Verification items for the finished model (mm, model axes). A direction names the side the tool comes from. Round coordinates to 2 decimals unless told otherwise and drop trailing zeros. Order: outer loops, then holes, each group sorted by start corner. A loop starts at its lowest first (then second) coordinate and runs counter-clockwise, first axis right, second up. Notation, with made-up numbers: M 46,6.5 L 66,6.5 A25 cw 66,22.5 Z; hole C 57,36 d8. An arc over 180 degrees is marked long. Use CSV: the item, a comma, the result in double quotes. Start each with the question number.
Q1. Sectioned sample at B-B (z = -4.25). Enter the section's corners in (x, y) (3 decimals), and give its area (3 significant figures).
Q2. Gauge pin test, flat ends, axial feed: pin 1 Ø2 at (y, z) = (231.5, -5.5) entering from -X; pin 2 Ø3 at (x, z) = (-5.5, -6.5) entering from +Y; pin 3 Ø3 at (x, z) = (-3, -4.5) entering from +Y. Record the tip position at first contact, or that the pin passes through.
Q3. Sectioned sample at C-C (y = 349.5). Enter the section's corners in (x, z).
Q4. Scan lines: line 1 (Y direction, x = 0, z = -1); line 2 (Y direction, x = -0.75, z = -4.25); line 3 (X direction, y = 276.5, z = -6). Record each from-to range of solid material in increasing order.
Q5. Sectioned sample at A-A (x = 0). Enter the section's corners in (y, z), and give its area (3 significant figures).
Q6. Mould release check, pull along Y, two halves, no side actions. Record for faces 1 (the face through (8.718, 232, -4)), 2 (the face through (7.218, 232, -4)): +Y half, -Y half, draft (parallel to the pull), parting line (faces both ways), or undercut.
Q7. Set-up check for faces 3 (the face through (-7, 237, 0)), 4 (the face through (0.14, -7.217, -3.735)): record each of +Z, -Z, +X, -X, +Y, -Y from which the full face is reachable in a straight line by a thin tool's end or side.
```python
from build123d import *

# Parameters (mm, degrees)
SKETCH3_W = 7.366
SKETCH3_H = 1.5


with BuildPart() as part:
    # Sweep1: sweep along a path in Sketch2
    with BuildLine(Plane.XY) as sweep1_path:
        Line((-7.217959412, 0.037533359), (-5.727035895, 286.753819557))
        ThreePointArc((-5.727035895, 286.753819557), (-5.72700281, 286.771488203), (-5.727087308, 286.789156677))
        Line((-5.727087308, 286.789156677), (-7.217819637, 470.60346355))
        ThreePointArc((-7.217819637, 470.60346355), (-0.029268466, 477.879997648), (7.218056998, 470.662))
        Line((7.218056998, 470.662), (7.218056998, 0))
        ThreePointArc((7.218056998, 0), (-0.018766743, -7.218032601), (-7.217959412, 0.037533359))
    # Sketch3 → Sweep1 (sweep)
    with BuildSketch(Plane(origin=(0, 0, 0), x_dir=(0, 0, -1), z_dir=(1, 0, 0))):
        with Locations((3.683, 478.630056998)):
            Rectangle(SKETCH3_W, SKETCH3_H)
    sweep(path=sweep1_path.line)


solid = part.part
```
Verdict:
1,outline,"M -8.718,0.045 A8.718 ccw 8.718,0 L 8.718,470.662 A8.718 ccw long -8.718,470.591 L -7.227,286.777 A1.155 cw -7.227,286.762 Z; hole M -7.218,0.038 A7.218 ccw 7.218,0 L 7.218,470.662 A7.218 ccw long -7.218,470.603 L -5.727,286.789 A2.655 cw -5.727,286.754 Z"
1,area,"1,490 mm²"
2,pin 1,"stops at x = -7.52"
2,pin 2,"stops at y = 478.41"
2,pin 3,"stops at y = 479.25"
3,outline,"M -7.74,-7.37 L -6.24,-7.37 L -6.24,0 L -7.74,0 Z; M 7.22,-7.37 L 8.72,-7.37 L 8.72,0 L 7.22,0 Z"
4,line 1,"y = -8.72 to -7.22, 477.88 to 479.38"
4,line 2,"y = -8.69 to -7.18, 477.84 to 479.35"
4,line 3,"x = -7.28 to -5.78, 7.22 to 8.72"
5,outline,"M -8.72,-7.37 L -7.22,-7.37 L -7.22,0 L -8.72,0 Z; M 477.88,-7.37 L 479.38,-7.37 L 479.38,0 L 477.88,0 Z"
5,area,"22.1 mm²"
6,face 1,"draft"
6,face 2,"undercut"
7,face 3,"+Z, +X, -X, +Y, -Y"
7,face 4,"+Z, -Z"
